Model file for the job. Use its own axes, mm. A direction names the side the tool comes from. Coordinates: 2 decimals unless noted, no trailing zeros. Write each loop counter-clockwise with the first axis right and the second up, starting at its lowest first coordinate (ties: lowest second). Pieces come first, ordered by that corner, then holes.
Q1. Band-saw the part on B-B, the plane y = 24. Write the cut outline in (x, z).
Q2. Pin check, flat tips, straight feed: P1, Ø1.6, axis at y = 2, z = 3, coming from the -X side; P2, Ø2, axis at y = 29.5, z = 11, coming from the -X side; P3, Ø5, axis at x = 34, y = 2, coming from the +Z side; P4, Ø1.9, axis at x = 12, y = 4, coming from the +Z side. Stop position of each tip, or through.
Q3. Which spindle directions (+Z, -Z, +X, -X, +Y, -Y) get a long thin tool onto all of the face, cutting with end or side? Do faces 1 (the flat face through (0, 23, 4)), 2 (the flat face through (32, 3, 4.762)). Say none if no direction does.
Q4. Band-saw the part on D-D, the plane x = 3. Write the cut outline in (y, z).
Q5. Pull direction X, two halves, no side cores. Call faces 3 (the cylindrical face through (1.91, 21.91, 10.89)), 4 (the flat face through (32, 3, 1.588)), 5 (the flat face through (22.536, 0.805, 0.783)): released by +X, released by -X, zero draft, split by the parting line, or undercut.
Q6. Band-saw the part on C-C, the plane z = 8.75. Write the cut outline in (x, y), plus the area to 3 significant figures.
Q7. Drill centre lines: probe 1 along X at (y, z) = (5, 2.75); probe 2 along Z at (x, y) = (18, 5); probe 3 along Y at (x, z) = (17, 3.5). Where is each one in solid material? Low to high.
Solid Edge part; units mm, degrees
sketch "Sketch1" plane through (0, 0, 0) normal (0, 0, 1) x (1, 0, 0)
  line L0 (0, 0) -> (44.45, 0)
  line L1 (44.45, 0) -> (44.45, 44.45)
  line L2 (44.45, 44.45) -> (0, 44.45)
  line L3 (0, 44.45) -> (0, 0)
  dimension "D1" = 44.45
  dimension "D2" = 44.45
extrude "Protrusion1" add sketch "Sketch1" along normal blind 12.7
fillet "Round_1" radius 6.35 4 edges at (22.225, 0, 12.7) (0, 22.225, 12.7) (22.225, 44.45, 12.7) (44.45, 22.225, 12.7)
sketch "Sketch2" plane through (22.225, 0, 3.175) normal (0, -1, 0) x (1, 0, 0)
  line L0 (14.2875, -1.5875) -> (4.7625, -1.5875)
  line L1 (4.7625, -1.5875) -> (4.7625, 1.5875)
  line L2 (4.7625, 1.5875) -> (14.2875, 1.5875)
  line L3 (14.2875, 1.5875) -> (14.2875, -1.5875)
  line L4 (-1.5875, -1.5875) -> (-14.2875, -1.5875)
  line L5 (-14.2875, -1.5875) -> (-14.2875, 1.5875)
  line L6 (-14.2875, 1.5875) -> (-1.5875, 1.5875)
  line L7 (-1.5875, 1.5875) -> (-1.5875, -1.5875)
  dimension "D1" = 1.5875
  dimension "D2" = 14.2875
  dimension "D3" = 1.5875
extrude "ExtrudedCutout_1" cut sketch "Sketch2" against normal blind 6.35
chamfer "Chamfer_1" distance 1.5875 angle 45 4 edges at (22.225, 0, 0) (0, 22.225, 0) (44.45, 22.225, 0) (22.225, 44.45, 0)
properties material "ABS Plastic, high impact"
Answer sheet:
1. outline: (0, 1.59) - (1.59, 0) - (42.86, 0) - (44.45, 1.59) - (44.45, 6.35) arc R6.35 ccw to (38.1, 12.7) - (6.35, 12.7) arc R6.35 ccw to (0, 6.35) - close
2. P1: stops at x = 0
2. P2: stops at x = 1.15
2. P3: stops at z = 12.42
2. P4: stops at z = 12.54
3. face 1: +Z, -Z, -X, +Y, -Y
3. face 2: -Y
4. outline: (0, 1.59) - (1.59, 0) - (42.86, 0) - (44.45, 1.59) - (44.45, 6.35) arc R6.35 ccw to (41.45, 11.74) - (3, 11.74) arc R6.35 ccw to (0, 6.35) - close
5. face 3: released by -X
5. face 4: undercut
5. face 5: zero draft
6. outline: (0.47, 0.47) - (43.98, 0.47) - (43.98, 43.98) - (0.47, 43.98) - close
6. area: 1,890 mm2
7. probe 1: x = 0 to 7.94, 20.64 to 26.99, 36.51 to 44.45
7. probe 2: z = 0 to 1.59, 4.76 to 12.55
7. probe 3: y = 6.35 to 44.45
